Geometry: final body of the model. Coordinates: model frame, mm. Face numbers are marked on the shaded views. A direction names the side the tool comes from. Give positions to 0.01 mm unless a question says otherwise; leave off trailing zeros. Write each loop counter-clockwise with the first axis right and the second up, starting at its lowest first coordinate (ties: lowest second). Pieces come first, ordered by that corner, then holes. Notation, with made-up numbers: (87.25, 20) - (122.25, 20) arc R12 cw to (122.25, 40) - close; hole circle Ø6 at (-9.5, -7). An arc over 180 degrees is marked (long way). Return JSON: item names as keys, results as strings.
from build123d import *

# Parameters (mm, degrees)
PAD_DEPTH       = 11
SKETCH001_R     = 2.55
POCKET_DEPTH    = 5
SKETCH002_R     = 1.3
POCKET001_DEPTH = 7
SKETCH003_R     = 1.3
POCKET002_DEPTH = 12
FILLET_R        = 0.3
FILLET001_R     = 0.3
FILLET002_R     = 0.3


with BuildPart() as part:
    # Sketch → Pad (new body)
    with BuildSketch(Plane.XY):
        Polygon((6.870468, 0), (3.435234, 5.95), (-3.435234, 5.95), (-6.870468, 0), (-3.435234, -5.95), (3.435234, -5.95), align=None)
    extrude(amount=PAD_DEPTH)

    # Sketch001 (on Face8 of Pad) → Pocket (cut)
    with BuildSketch(Plane.XY.offset(11)):
        Circle(SKETCH001_R)
    extrude(amount=-POCKET_DEPTH, mode=Mode.SUBTRACT)

    # Sketch002 (on Face4 of Pocket) → Pocket001 (cut)
    with BuildSketch(Plane(origin=(0, 0, 0), x_dir=(1, 0, 0), z_dir=(0, 0, -1))):
        Circle(SKETCH002_R)
    extrude(amount=-POCKET001_DEPTH, mode=Mode.SUBTRACT)

    # Sketch003 (on Face6 of Pocket001) → Pocket002 (cut)
    with BuildSketch(Plane.XZ.offset(5.95)):
        with Locations((0, 8)):
            Circle(SKETCH003_R)
    extrude(amount=-POCKET002_DEPTH, mode=Mode.SUBTRACT)

    # Fillet
    fillet_edges = [part.edges().sort_by_distance(p)[0] for p in [
        (5.152851, -2.975, 11),
        (0, -5.95, 11),
        (-5.152851, -2.975, 11),
        (-5.152851, 2.975, 11),
        (0, 5.95, 11),
        (5.152851, 2.975, 11),
    ]]
    fillet(fillet_edges, radius=FILLET_R)

    # Fillet001
    fillet001_edges = [part.edges().sort_by_distance(p)[0] for p in [
        (0, 5.95, 0),
        (-5.152851, 2.975, 0),
        (-5.152851, -2.975, 0),
        (0, -5.95, 0),
        (5.152851, -2.975, 0),
        (5.152851, 2.975, 0),
    ]]
    fillet(fillet001_edges, radius=FILLET001_R)

    # Fillet002
    fillet002_edges = [part.edges().sort_by_distance(p)[0] for p in [
        (3.435234, -5.95, 5.5),
        (6.870468, 0, 5.5),
        (-3.435234, -5.95, 5.5),
        (-6.870468, 0, 5.5),
        (-3.435234, 5.95, 5.5),
        (3.435234, 5.95, 5.5),
    ]]
    fillet(fillet002_edges, radius=FILLET002_R)


solid = part.part
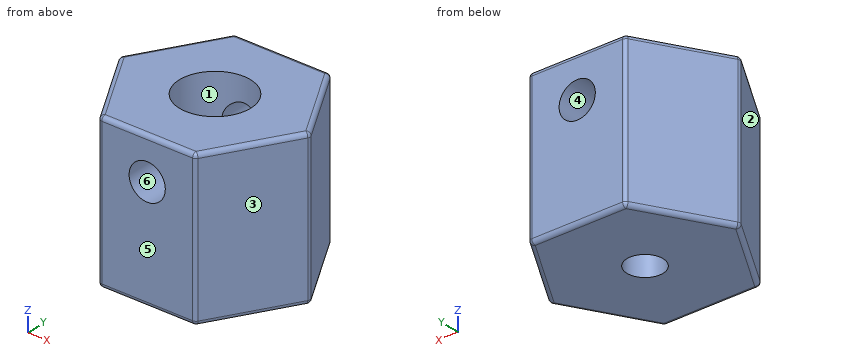
Q1. Material intervals for probe 1 along Z at (x, y) = (0, 3.55); probe 2 along X at (y, z) = (-0.5, 6.75); probe 3 along X at (y, z) = (-4.55, 8), sorted ascending. Write a range as [from, to].
Answer key:
{"probe 1": "z = [0, 6.7], [9.3, 11]", "probe 2": "x = [-6.58, -2.5], [2.5, 6.58]", "probe 3": "x = [-4.24, -1.3], [1.3, 4.24]"}
Q2. Pin query (flat end, axial travel): P1, Ø4, axis at y = -2.5, z = 4.5, coming from the +X side; P2, Ø4, axis at x = 0, y = 0, coming from the +Z side; P3, Ø5, axis at y = -3, z = 6, coming from the -X side. Return the tip coordinate at first contact, or that it passes through.
Answer key:
{"P1": "stops at x = 6.58", "P2": "stops at z = 6", "P3": "stops at x = -6.58"}
Q3. Section query C-C, the plane z = 9.5. Return the cut outline in (x, y), plus the area to 3 significant figures.
Answer key:
{"outline": "(-6.78, -0.15) - (-3.52, -5.8) arc R0.3 ccw to (-3.26, -5.95) - (3.26, -5.95) arc R0.3 ccw to (3.52, -5.8) - (6.78, -0.15) arc R0.3 ccw to (6.78, 0.15) - (3.52, 5.8) arc R0.3 ccw to (3.26, 5.95) - (-3.26, 5.95) arc R0.3 ccw to (-3.52, 5.8) - (-6.78, 0.15) arc R0.3 ccw to start; hole circle Ø5.1 at (0, 0)", "area": "102 mm^2"}
Q4. Section query A-A, the plane x = 0. Return the cut outline in (y, z), plus the area to 3 significant figures.
Answer key:
{"outline": "(-5.95, 0.3) arc R0.3 ccw to (-5.65, 0) - (-1.3, 0) - (-1.3, 6) - (-2.55, 6) - (-2.55, 6.7) - (-5.95, 6.7) - close; (-5.95, 9.3) - (-2.55, 9.3) - (-2.55, 11) - (-5.65, 11) arc R0.3 ccw to (-5.95, 10.7) - close; (1.3, 0) - (5.65, 0) arc R0.3 ccw to (5.95, 0.3) - (5.95, 6.7) - (2.55, 6.7) - (2.55, 6) - (1.3, 6) - close; (2.55, 9.3) - (5.95, 9.3) - (5.95, 10.7) arc R0.3 ccw to (5.65, 11) - (2.55, 11) - close", "area": "72.0 mm^2"}
Q5. Section query D-D, the plane z = 2.5. Return the cut outline in (x, y).
Answer key:
{"outline": "(-6.78, -0.15) - (-3.52, -5.8) arc R0.3 ccw to (-3.26, -5.95) - (3.26, -5.95) arc R0.3 ccw to (3.52, -5.8) - (6.78, -0.15) arc R0.3 ccw to (6.78, 0.15) - (3.52, 5.8) arc R0.3 ccw to (3.26, 5.95) - (-3.26, 5.95) arc R0.3 ccw to (-3.52, 5.8) - (-6.78, 0.15) arc R0.3 ccw to start; hole circle Ø2.6 at (0, 0)"}
Q6. Mould query, pull axis X, two halves, no side actions, for the marked faces 3, 4, 5 and 6. Classes: pulls with the +X half, pulls with the -X half, needs draft (parallel to the pull), parting line crosses it, or undercut.
Answer key:
{"face 3": "pulls with the +X half", "face 4": "undercut", "face 5": "needs draft", "face 6": "undercut"}
Q7. Section query B-B, the plane z = 8. Return the cut outline in (x, y), plus the area to 3 significant figures.
Answer key:
{"outline": "(-6.78, -0.15) - (-3.52, -5.8) arc R0.3 ccw to (-3.26, -5.95) - (-1.3, -5.95) - (-1.3, -2.19) arc R2.55 cw to (-1.3, 2.19) - (-1.3, 5.95) - (-3.26, 5.95) arc R0.3 ccw to (-3.52, 5.8) - (-6.78, 0.15) arc R0.3 ccw to start; (1.3, -5.95) - (3.26, -5.95) arc R0.3 ccw to (3.52, -5.8) - (6.78, -0.15) arc R0.3 ccw to (6.78, 0.15) - (3.52, 5.8) arc R0.3 ccw to (3.26, 5.95) - (1.3, 5.95) - (1.3, 2.19) arc R2.55 cw to (1.3, -2.19) - close", "area": "83.9 mm^2"}
Q8. Set-up query: the marked faces 1 and 2. Return all of +Z, -Z, +X, -X, +Y, -Y with unobstructed straight access to the full face (end or side cutting, diameter ignored); none if empty.
Answer key:
{"face 1": "+Z", "face 2": "+Z, -Z, -X, -Y"}
